Verification items for the finished model (mm, model axes). Face numbers are marked on the shaded views. A direction names the side the tool comes from. Round coordinates to 2 decimals unless told otherwise and drop trailing zeros. Loops run counter-clockwise (first coordinate to the right, second up) from the corner with the lowest first, then second, coordinate; pieces in that order, holes last. Notation, with made-up numbers: (14.25, -14.5) -> (66.25, -14.5) arc R24 cw to (66.25, 11.5) -> close; hole circle Ø5 at (14.5, 44). An arc over 180 degrees is marked (long way). Use CSV: the item, a comma, the result in double quotes. Start each with the question number.
```python
from build123d import *

# Parameters (mm, degrees)
SKETCH1_W           = 55
SKETCH1_H           = 55
SKETCH1_R           = 1.75
BOSS_EXTRUDE1_DEPTH = 10
SKETCH2_R           = 15
CUT_EXTRUDE1_DEPTH  = 41.155946011
SKETCH3_R           = 1.5
CUT_EXTRUDE2_DEPTH  = 41.155946011
SKETCH4_R           = 3.25
CUT_EXTRUDE3_DEPTH  = 6
CHAMFER1_SIZE       = 5


with BuildPart() as part:
    # Sketch1 → Boss-Extrude1 (new body)
    with BuildSketch(Plane.XY):
        Rectangle(SKETCH1_W, SKETCH1_H)
        with Locations((19.445436483, 19.445436483)):
            Circle(SKETCH1_R, mode=Mode.SUBTRACT)
        with Locations((-19.445436483, 19.445436483)):
            Circle(SKETCH1_R, mode=Mode.SUBTRACT)
        with Locations((-19.445436483, -19.445436483)):
            Circle(SKETCH1_R, mode=Mode.SUBTRACT)
        with Locations((19.445436483, -19.445436483)):
            Circle(SKETCH1_R, mode=Mode.SUBTRACT)
    extrude(amount=BOSS_EXTRUDE1_DEPTH)

    # Sketch2 → Cut-Extrude1 (cut, through all)
    with BuildSketch(Plane(origin=(0, 0, 0), x_dir=(-1, 0, 0), z_dir=(0, 0, -1))):
        Circle(SKETCH2_R)
    extrude(amount=-CUT_EXTRUDE1_DEPTH, mode=Mode.SUBTRACT)

    # Sketch3 → Cut-Extrude2 (cut, through all)
    with BuildSketch(Plane(origin=(0, 0, 0), x_dir=(-1, 0, 0), z_dir=(0, 0, -1))):
        with Locations((0, 21.920310217)):
            Circle(SKETCH3_R)
        with Locations((21.920310217, 0)):
            Circle(SKETCH3_R)
        with Locations((0, -21.920310217)):
            Circle(SKETCH3_R)
        with Locations((-21.920310217, 0)):
            Circle(SKETCH3_R)
    extrude(amount=-CUT_EXTRUDE2_DEPTH, mode=Mode.SUBTRACT)

    # Sketch4 → Cut-Extrude3 (cut)
    with BuildSketch(Plane(origin=(0, 0, 0), x_dir=(-1, 0, 0), z_dir=(0, 0, -1))):
        with Locations((0, 21.920310217)):
            Circle(SKETCH4_R)
        with Locations((21.920310217, 0)):
            Circle(SKETCH4_R)
        with Locations((0, -21.920310217)):
            Circle(SKETCH4_R)
        with Locations((-21.920310217, 0)):
            Circle(SKETCH4_R)
    extrude(amount=-CUT_EXTRUDE3_DEPTH, mode=Mode.SUBTRACT)

    # Chamfer1
    chamfer1_edges = [part.edges().sort_by_distance(p)[0] for p in [
        (27.5, -27.5, 5),
        (-27.5, -27.5, 5),
        (-27.5, 27.5, 5),
        (27.5, 27.5, 5),
    ]]
    chamfer(chamfer1_edges, length=CHAMFER1_SIZE)


solid = part.part
```
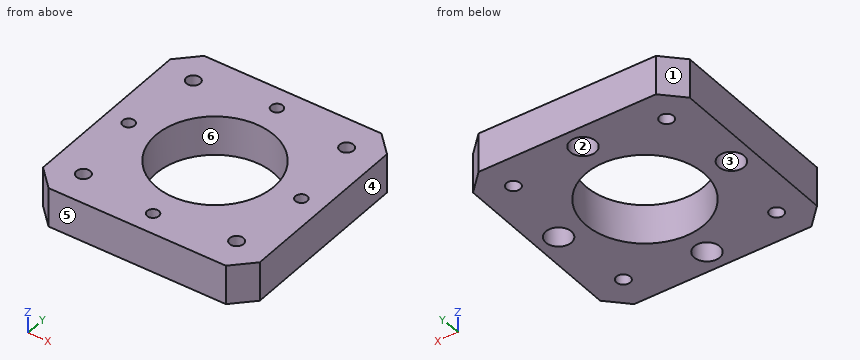
Q1. Tool access check on the marked faces 1 and 2. Record the directions out of +Z, -Z, +X, -X, +Y, -Y that give a thin tool (end or side, any length) a straight path to the whole face; none if there is none.
Q2. Depth check by flat-ended pin: pin 1 Ø6 at (x, y) = (-21.92, 0) entering from -Z. Enter the tip coordinate at first touch or a pass-through.
Q3. Cross-section at C-C (y = 12). Record the boundary of the cut face in (x, z).
Q4. Release check for a two-part mould opening along Y. For the marked faces 3, 4, 5 and 6 record: +Y half, -Y half, draft (parallel to the pull), parting line (faces both ways), or undercut.
Q5. Thickness scan on L1, parallel to Y at x = 0, z = 4.55; L2, parallel to Y at x = 0, z = 7.5; L3, parallel to X at y = 22, z = 4.25. Record the ranges inside material, lowest first. Write a range as from..to.
Q6. Cross-section at A-A (y = 0). Record the boundary of the cut face in (x, z), and give its area (3 significant figures).
Q7. Cross-section at B-B (x = -9). Record the boundary of the cut face in (y, z).
Answer list:
1,face 1,"+Z, -Z, -X, +Y"
1,face 2,"-Z"
2,pin 1,"stops at z = 6"
3,outline,"(-27.5, 0) -> (-9, 0) -> (-9, 10) -> (-27.5, 10) -> close; (9, 0) -> (27.5, 0) -> (27.5, 10) -> (9, 10) -> close"
4,face 3,"undercut"
4,face 4,"draft"
4,face 5,"-Y half"
4,face 6,"undercut"
5,L1,"y = -27.5..-25.17, -18.67..-15, 15..18.67, 25.17..27.5"
5,L2,"y = -27.5..-23.42, -20.42..-15, 15..20.42, 23.42..27.5"
5,L3,"x = -27.5..-3.25, 3.25..27.5"
6,outline,"(-27.5, 0) -> (-25.17, 0) -> (-25.17, 6) -> (-23.42, 6) -> (-23.42, 10) -> (-27.5, 10) -> close; (-20.42, 6) -> (-18.67, 6) -> (-18.67, 0) -> (-15, 0) -> (-15, 10) -> (-20.42, 10) -> close; (15, 0) -> (18.67, 0) -> (18.67, 6) -> (20.42, 6) -> (20.42, 10) -> (15, 10) -> close; (23.42, 6) -> (25.17, 6) -> (25.17, 0) -> (27.5, 0) -> (27.5, 10) -> (23.42, 10) -> close"
6,area,"148 mm2"
7,outline,"(-27.5, 0) -> (-12, 0) -> (-12, 10) -> (-27.5, 10) -> close; (12, 0) -> (27.5, 0) -> (27.5, 10) -> (12, 10) -> close"
